Verification items for the finished model (mm, model axes). Face numbers are marked on the shaded views. A direction names the side the tool comes from. Give positions to 0.01 mm unless a question says otherwise; leave off trailing zeros. Order: outer loops, then holes, each group sorted by start corner. A loop starts at its lowest first (then second) coordinate and runs counter-clockwise, first axis right, second up. Notation, with made-up numbers: M 8.25,13.5 L 39.25,13.5 A8 cw 39.25,24.5 Z; hole C -8,-39.5 d2. An arc over 180 degrees is marked long. Answer as a JSON object with one key per item and string values.
Autodesk Inventor part; units mm, degrees
ref_plane "YZ Plane" through (0, 0, 0) normal (1, 0, 0) x (0, 1, 0)
ref_plane "XZ Plane" through (0, 0, 0) normal (0, 1, 0) x (-1, 0, 0)
ref_plane "XY Plane" through (0, 0, 0) normal (0, 0, 1) x (1, 0, 0)
sketch "Sketch1" plane through (0, 0, 0) normal (0, 1, 0) x (-1, 0, 0)
  line L0 (-51, 98.425) -> (51, 98.425)
  line L1 (51, 98.425) -> (51, -98.425)
  line L2 (51, -98.425) -> (-51, -98.425)
  line L3 (-51, -98.425) -> (-51, 98.425)
  line L4 (-51, 98.425) -> (51, -98.425) construction
  line L5 (51, 98.425) -> (-51, -98.425) construction
  point P0 (0, 0)
  dimension "d0" = 102
  dimension "d1" = 196.85
extrude "Extrusion1" add sketch "Sketch1" along normal blind 6
sketch "Sketch2" plane through (0, 6, 0) normal (0, 1, 0) x (1, 0, 0)
  line L0 (51, -88.9) -> (-51, -88.9)
  line L1 (-51, -88.9) -> (-51, 88.9)
  line L2 (-51, 88.9) -> (51, 88.9)
  line L3 (51, 88.9) -> (51, -88.9)
  line L4 (51, -88.9) -> (-51, 88.9) construction
  line L5 (-51, -88.9) -> (51, 88.9) construction
  point P0 (0, 0)
  dimension "d4" = 102
  dimension "d5" = 177.8
extrude "Extrusion2" add sketch "Sketch2" along normal blind 56
draft "FaceDraft1" angle 15 pull direction (0, 1, 0) faces at (17, 24.6667, 88.9) fixed edges at (0, 6, 88.9)
draft "FaceDraft2" angle 15 pull direction (0, 1, 0) faces at (-17, 24.6667, -88.9) fixed edges at (0, 6, -88.9)
sketch "Sketch3" plane through (0, 0, 0) normal (0, -1, 0) x (1, 0, 0)
  line L0 (32.4713, 98.425) -> (27.4713, 98.425)
  line L1 (27.4713, 98.425) -> (27.4713, 90.925)
  line L2 (27.4713, 90.925) -> (32.4713, 90.925)
  line L3 (32.4713, 90.925) -> (32.4713, 98.425)
  line L4 (32.4713, 98.425) -> (27.4713, 90.925) construction
  line L5 (27.4713, 98.425) -> (32.4713, 90.925) construction
  line L6 (51, -98.425) -> (51, 98.425)
  line L7 (-51, 98.425) -> (51, 98.425)
  line L8 (-27.4727, 90.925) -> (-32.4727, 90.925)
  line L9 (-32.4727, 90.925) -> (-32.4727, 98.425)
  line L10 (-32.4727, 98.425) -> (-27.4727, 98.425)
  line L11 (-27.4727, 98.425) -> (-27.4727, 90.925)
  line L12 (-27.4727, 90.925) -> (-32.4727, 98.425) construction
  line L13 (-32.4727, 90.925) -> (-27.4727, 98.425) construction
  line L14 (-51, 98.425) -> (-51, -98.425)
  line L15 (51, 0) -> (-51, 0)
  line L16 (-51, -73.8948) -> (-51, 73.8948)
  line L17 (32.4713, -98.425) -> (27.4713, -98.425)
  line L18 (27.4713, -98.425) -> (27.4713, -90.925)
  line L19 (27.4713, -90.925) -> (32.4713, -90.925)
  line L20 (32.4713, -90.925) -> (32.4713, -98.425)
  line L21 (-27.4727, -90.925) -> (-32.4727, -90.925)
  line L22 (-32.4727, -90.925) -> (-32.4727, -98.425)
  line L23 (-32.4727, -98.425) -> (-27.4727, -98.425)
  line L24 (-27.4727, -98.425) -> (-27.4727, -90.925)
  point P0 (0, 0)
  point P1 (29.9713, 94.675)
  point P2 (-29.9727, 94.675)
  point P3 (29.9713, -94.675)
  dimension "d10" = 5
  dimension "d11" = 7.5
  dimension "d12" = 21.0287
  dimension "d13" = 7.5
  dimension "d14" = 5
  dimension "d16" = 59.944
  dimension "d17" = 0
extrude "Extrusion3" cut sketch "Sketch3" against normal blind 56 contours L3 L2 L1 L0 | L11 L8 L9 L7 | L17 L18 L19 L20 | L24 L23 L22 L21
fillet "Fillet1" radius 2.159 20 edges at (27.4713, 3, 90.925) (32.4713, 3, 90.925) (32.4713, 3, 98.425) (27.4713, 3, 98.425) (-27.4727, 3, 90.925) (-32.4727, 3, 90.925) (-32.4727, 3, 98.425) (-27.4727, 3, 98.425) (-27.4727, 3, -98.425) (-27.4727, 3, -90.925) (-32.4727, 3, -90.925) (-32.4727, 3, -98.425) (27.4713, 3, -90.925) (27.4713, 3, -98.425) (32.4713, 3, -90.925) (32.4713, 3, -98.425) (51, 3, -98.425) (-51, 3, -98.425) (-51, 3, 98.425) (51, 3, 98.425)
sketch "Sketch4" plane through (51, 62, 73.8948) normal (1, 0, 0) x (0, 0, -1)
  line L0 (41.3948, -25) -> (106.3948, -25)
  line L1 (106.3948, -25) -> (106.3948, -10)
  line L2 (106.3948, -10) -> (41.3948, -10)
  line L3 (41.3948, -10) -> (41.3948, -25)
  line L4 (41.3948, -25) -> (106.3948, -10) construction
  line L5 (106.3948, -25) -> (41.3948, -10) construction
  line L6 (0, 0) -> (147.7897, 0)
  circle A0 centre (136.9784, -42.8226) radius 6.25
  point P0 (73.8948, -62)
  point P1 (73.8948, -17.5)
  dimension "d21" = 65
  dimension "d22" = 15
  dimension "d23" = 17.5
  dimension "d24" = 12.5
extrude "Extrusion4" add sketch "Sketch4" along normal blind 15
equation "\"d13\" = d11"
equation "\"d14\" = d10"
properties part number "12v_dc_to_dc"
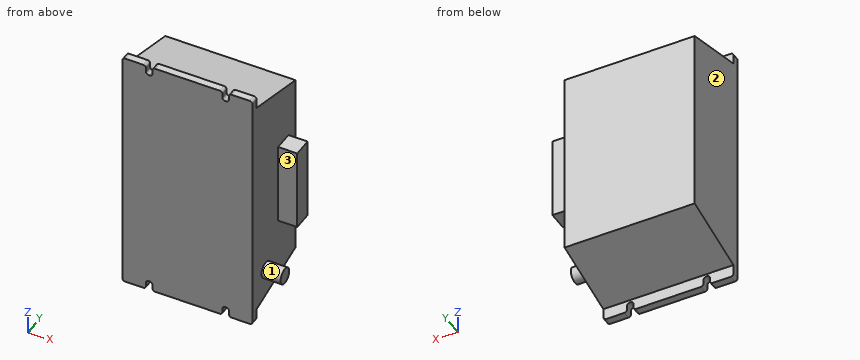
Q1. Section check C-C on z = 65.5. Record the cut outline in (x, y).
Resolved:
{"outline": "M -51,0 L 51,0 L 51,62 L -51,62 Z"}
Q2. Material ranges on L1, parallel to X at y = 18.5, z = -77; L2, parallel to Z at x = 60.5, y = 19; L3, parallel to Z at x = -45, y = 39.5, recorded low to high.
Resolved:
{"L1": "x = -51 to 51", "L2": "z = -69.33 to -56.84", "L3": "z = -79.92 to 79.92"}
Q3. Section check A-A on z = 7. Record the cut outline in (x, y), then the cut area to 3 significant figures.
Resolved:
{"outline": "M -51,0 L 51,0 L 51,37 L 66,37 L 66,52 L 51,52 L 51,62 L -51,62 Z", "area": "6,550 mm²"}
Q4. Gauge pin test, flat ends, axial feed: pin 1 Ø5 at (x, y) = (8.5, 17.5) entering from -Z; pin 2 Ø3 at (x, z) = (17, -92.5) entering from +Y; pin 3 Ø0.5 at (x, y) = (30, 3.5) entering from -Z (3 decimals). Record the tip position at first contact, or that the pin passes through.
Resolved:
{"pin 1": "stops at z = -86.49", "pin 2": "stops at y = 6", "pin 3": "stops at z = -90.925"}
Q5. Section check B-B on x = -22.5. Record the cut outline in (y, z) (3 decimals).
Resolved:
{"outline": "M 0,-98.425 L 6,-98.425 L 6,-88.9 L 62,-73.895 L 62,73.895 L 6,88.9 L 6,98.425 L 0,98.425 Z"}
Q6. Section check D-D on y = 10.5. Record the cut outline in (x, z), then the cut area to 3 significant figures.
Resolved:
{"outline": "M -51,-87.69 L 51,-87.69 L 51,87.69 L -51,87.69 Z", "area": "17,900 mm²"}
Q7. Tool access check on the marked faces 1, 2 and 3. Record the directions out of +Z, -Z, +X, -X, +Y, -Y that give a thin tool (end or side, any length) a straight path to the whole face; none if there is none.
Resolved:
{"face 1": "+X", "face 2": "+Z, -Z, -X, +Y, -Y", "face 3": "+Z, -Z, +X, -Y"}
